Part model, mm, in its own coordinate system. Face numbers are marked on the shaded views. A direction names the side the tool comes from. Round coordinates to 2 decimals unless told otherwise and drop trailing zeros. Loops run counter-clockwise (first coordinate to the right, second up) from the corner with the lowest first, then second, coordinate; pieces in that order, holes last. Notation, with made-up numbers: (-27, -10) - (-5, -10) arc R32 cw to (-5, 26) - close; hole circle Ø3 at (33, 63). An arc over 180 degrees is marked (long way). Put each result on its own line as item: value.
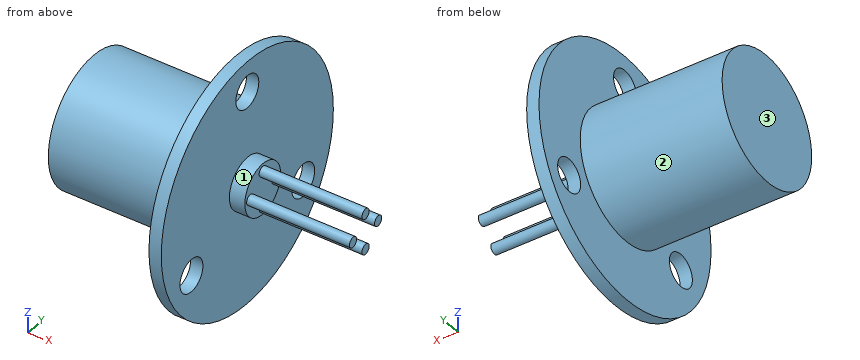
from build123d import *

# Parameters (mm, degrees)
CROQUIS1_W              = 13.8
CROQUIS1_H              = 6.25
CROQUIS1_W_2            = 1.5
CROQUIS1_H_2            = 2.5
CROQUIS2_R              = 1.6
CORTAR_EXTRUIR1_DEPTH   = 3.2
MATRIZC1_COUNT          = 3
CROQUIS3_R              = 0.5
SALIENTE_EXTRUIR1_DEPTH = 10
MATRIZC2_COUNT          = 4


with BuildPart() as part:
    # Croquis1 → Revolución1 (revolve)
    with BuildSketch(Plane(origin=(0, 0, 0), x_dir=(-1, 0, 0), z_dir=(0, 1, 0))):
        with Locations((-6.9, 3.125)):
            Rectangle(CROQUIS1_W, CROQUIS1_H)
        Polygon((-15, 0), (-13.8, 0), (-13.8, 6.25), (-13.8, 12), (-15, 12), (-15, 2.5), align=None)
        with Locations((-15.75, 1.25)):
            Rectangle(CROQUIS1_W_2, CROQUIS1_H_2)
    revolve(axis=Axis((0, 0, 0), (1, 0, 0)))

    # Croquis2 → Cortar-Extruir1 (cut)
    with BuildSketch(Plane.YZ.offset(15)):
        with Locations(Location((0, 9, 0), (0, 0, 270))):
            Circle(CROQUIS2_R)
    cortar_extruir1 = extrude(amount=-CORTAR_EXTRUIR1_DEPTH, mode=Mode.SUBTRACT)

    # MatrizC1: Cortar-Extruir1 ×3 about axis
    matrizc1_axis = Axis((0, 0, 0), (1, 0, 0))
    for i in range(1, MATRIZC1_COUNT):
        add(cortar_extruir1.rotate(matrizc1_axis, i * 360 / MATRIZC1_COUNT), mode=Mode.SUBTRACT)

    # Croquis3 → Saliente-Extruir1 (add)
    with BuildSketch(Plane.YZ.offset(16.5)):
        with Locations(Location((0, 1.75, 0), (0, 0, 270))):
            Circle(CROQUIS3_R)
    saliente_extruir1 = extrude(amount=SALIENTE_EXTRUIR1_DEPTH)

    # MatrizC2: Saliente-Extruir1 ×4 about axis
    matrizc2_axis = Axis((0, 0, 0), (1, 0, 0))
    for i in range(1, MATRIZC2_COUNT):
        add(saliente_extruir1.rotate(matrizc2_axis, i * 360 / MATRIZC2_COUNT))


solid = part.part
1. Band-saw the part on C-C (x = 22.25). List the corners of the cut face in (y, z), plus the area to 3 significant figures.
A:
outline: circle Ø1 at (-1.75, 0); circle Ø1 at (0, -1.75); circle Ø1 at (0, 1.75); circle Ø1 at (1.75, 0)
area: 3.14 mm²
2. Pin check, flat tips, straight feed: P1, Ø4, axis at y = 1, z = 4.5, coming from the +X side; P2, Ø8, axis at x = 14, y = -9, coming from the +Z side; P3, Ø4, axis at x = 23.5, y = -1.5, coming from the +Z side; P4, Ø2.5, axis at y = 7.79, z = -4.5, coming from the +X side. Stop position of each tip, or through.
A:
P1: stops at x = 15
P2: stops at z = 10.91
P3: stops at z = 2.25
P4: passes through
3. Probe line 1 along Y through (x, z) = (14.1, -4.5); line 2 along X through (y, z) = (-2.75, -7.75); line 3 along X through (y, z) = (-1, 3). List the from-to ranges inside material, lowest first. Write a range as [from, to].
A:
line 1: y = [-11.12, -9.39], [-6.19, 6.19], [9.39, 11.12]
line 2: x = [13.8, 15]
line 3: x = [0, 15]
4. Band-saw the part on B-B (z = 0). List the corners of the cut face in (x, y), plus the area to 3 significant figures.
A:
outline: (0, -6.25) - (13.8, -6.25) - (13.8, -12) - (15, -12) - (15, -2.5) - (16.5, -2.5) - (16.5, -2.25) - (26.5, -2.25) - (26.5, -1.25) - (16.5, -1.25) - (16.5, 1.25) - (26.5, 1.25) - (26.5, 2.25) - (16.5, 2.25) - (16.5, 2.5) - (15, 2.5) - (15, 12) - (13.8, 12) - (13.8, 6.25) - (0, 6.25) - close
area: 229 mm²
5. Band-saw the part on D-D (y = -3). List the corners of the cut face in (x, z).
A:
outline: (0, -5.48) - (13.8, -5.48) - (13.8, -11.62) - (15, -11.62) - (15, 11.62) - (13.8, 11.62) - (13.8, 5.48) - (0, 5.48) - close
6. Band-saw the part on A-A (y = 0). List the corners of the cut face in (x, z).
A:
outline: (0, -6.25) - (13.8, -6.25) - (13.8, -12) - (15, -12) - (15, -2.5) - (16.5, -2.5) - (16.5, -2.25) - (26.5, -2.25) - (26.5, -1.25) - (16.5, -1.25) - (16.5, 1.25) - (26.5, 1.25) - (26.5, 2.25) - (16.5, 2.25) - (16.5, 2.5) - (15, 2.5) - (15, 7.4) - (13.8, 7.4) - (13.8, 6.25) - (0, 6.25) - close; (13.8, 10.6) - (15, 10.6) - (15, 12) - (13.8, 12) - close
7. Tool access for the marked faces 1, 2 and 3: list every direction of +Z, -Z, +X, -X, +Y, -Y with a clear straight run to the whole face (end or side of a thin tool).
A:
face 1: +X
face 2: -X
face 3: +Z, -Z, -X, +Y, -Y
